Autodesk Inventor part; units mm, degrees
ref_plane "YZ Plane" through (0, 0, 0) normal (1, 0, 0) x (0, 1, 0)
ref_plane "XZ Plane" through (0, 0, 0) normal (0, 1, 0) x (-1, 0, 0)
ref_plane "XY Plane" through (0, 0, 0) normal (0, 0, 1) x (1, 0, 0)
sketch "Эскиз1" plane through (0, 0, 0) normal (0, 1, 0) x (-1, 0, 0)
  circle A0 centre (15.0247, -0.005) radius 9.5
  circle A1 centre (0.0247, 14.995) radius 9.5
  circle A2 centre (0.0247, -15.005) radius 9.5
  arc A3 (-4.923, -24.5094) -> (-4.9258, 24.5) centre (0.0275, -0.0044) ccw
  arc A4 (-13.7779, 22.8932) -> (-4.9258, 24.5) centre (-49.9753, 247.495) ccw
  line L0 (-13.7779, 22.8932) -> (-13.7779, -22.9031)
  arc A5 (-4.923, -24.5094) -> (-4.9258, 24.5) centre (0.0275, -0.0044) ccw
  circle A6 centre (15.0247, -0.005) radius 9.5
  circle A7 centre (0.0247, 14.995) radius 9.5
  circle A8 centre (0.0247, -15.005) radius 9.5
  arc A9 (-4.923, -24.5094) -> (-4.9258, 24.5) centre (0.0275, -0.0044) ccw
  arc A10 (-13.7779, 22.8932) -> (-4.9258, 24.5) centre (-49.9753, 247.495) ccw
  arc A11 (-4.923, -24.5094) -> (-13.7779, -22.9031) centre (-49.9479, -247.5094) ccw
  line L1 (-13.7779, 22.8932) -> (-13.7779, -22.9031)
  arc A12 (-4.923, -24.5094) -> (-4.9258, 24.5) centre (0.0275, -0.0044) ccw
  line L2 (0.0275, -25.0044) -> (-13.7779, -25.0044)
  line L3 (-13.7779, -25.0044) -> (-13.7779, -22.9031)
  line L4 (0.0275, 24.9956) -> (-13.7779, 24.9956)
  line L5 (-13.7779, 24.9956) -> (-13.7779, 22.8932)
  point P0 (0, 0)
extrude "Выдавливание1" add sketch "Эскиз1" along normal blind 6
sketch "Эскиз2" plane through (0, 6, 0) normal (0, 1, 0) x (1, 0, 0)
  line L0 (0, 0) -> (10, 0)
  circle A0 centre (10, 0) radius 2.1
  line L1 (0, 0) -> (-14.1421, -14.1421)
  line L2 (0, 0) -> (20, 0) construction
  line L3 (0, 0) -> (-14.1421, 14.1421)
  circle A1 centre (-14.1421, -14.1421) radius 2.1
  circle A2 centre (-14.1421, 14.1421) radius 2.1
  dimension "d2" = 10
  dimension "d3" = 4.2
  dimension "d4" = 20
  dimension "d5" = 135
  dimension "d6" = 20
  dimension "d7" = 90
  dimension "d8" = 4.2
  dimension "d9" = 4.2
extrude "Выдавливание2" cut sketch "Эскиз2" against normal blind 15.25
equation "\"d3\" = d9"
equation "\"d8\" = d9"
properties part number "000.403 -  Прижим подшипников"
The listing builds one solid part. Answer for the finished solid, in the listing's coordinates (mm). Coordinates: 2 decimals unless noted, no trailing zeros. Write each loop counter-clockwise with the first axis right and the second up, starting at its lowest first coordinate (ties: lowest second). Pieces come first, ordered by that corner, then holes.
Q1. Section C-C, the plane x = -6.5 is taken. Write down the section's boundary in (y, z).
Returned:
outline: (0, -24.15) - (6, -24.15) - (6, -21.96) - (0, -21.96) - close; (0, -8.05) - (6, -8.05) - (6, -4.2) - (0, -4.2) - close; (0, 4.19) - (6, 4.19) - (6, 8.04) - (0, 8.04) - close; (0, 21.95) - (6, 21.95) - (6, 24.14) - (0, 24.14) - close
Q2. The mould has two halves that part along X. Classify faces 1 (the flat face through (7, 3, 24.996)), 2 (the cylindrical face through (-14.415, 3.042, -16.224)), 3 (the cylindrical face through (-25.02, 2.96, 0.55)): released by +X, released by -X, zero draft, split by the parting line, or undercut.
Returned:
face 1: zero draft
face 2: undercut
face 3: released by -X
Q3. Section D-D, the plane y = 1.95 is taken. Write down the section's boundary in (x, z) (1 decimal).
Returned:
outline: (0, -25) - (13.8, -25) - (13.8, 25) - (0, 25) arc R25 ccw to start; hole circle Ø19 at (-15, 0); hole circle Ø4.2 at (-14.1, -14.1); hole circle Ø4.2 at (-14.1, 14.1); hole circle Ø19 at (0, -15); hole circle Ø19 at (0, 15); hole circle Ø4.2 at (10, 0)
Q4. Section B-B, the plane z = -3.5 is taken. Write down the section's boundary in (x, y), then the cut area to 3 significant figures.
Returned:
outline: (-24.78, 0) - (-23.86, 0) - (-23.86, 6) - (-24.78, 6) - close; (-6.19, 0) - (13.78, 0) - (13.78, 6) - (-6.19, 6) - close
area: 125 mm2
Q5. Given P1, Ø1, axis at y = 5.5, z = -17, coming from the -X side; P2, Ø2, axis at x = -3.5, y = 1, coming from the +Z side, each flat-ended and moving along its own axis, determine where each tip first touches the part or whether it passes through.
Returned:
P1: stops at x = -18.81
P2: stops at z = 24.87
Q6. Find the intervals of material crossed by line 1 along X through (y, z) = (1.65, 8.5); line 2 along X through (y, z) = (4.05, 0); line 3 along Z through (x, y) = (-15, 3.75), in increasing order.
Returned:
line 1: x = -23.54 to -19.26, -10.79 to -6.96, 6.91 to 13.78
line 2: x = -25.03 to -24.52, -5.52 to 7.9, 12.1 to 13.78
line 3: z = -20.03 to -16.06, -12.23 to -9.5, 9.49 to 12.23, 16.06 to 20.02
Q7. Section A-A, the plane x = 10 is taken. Write down the section's boundary in (y, z), then the cut area to 3 significant figures.
Returned:
outline: (0, -25) - (6, -25) - (6, -2.1) - (0, -2.1) - close; (0, 2.1) - (6, 2.1) - (6, 25) - (0, 25) - close
area: 275 mm2
